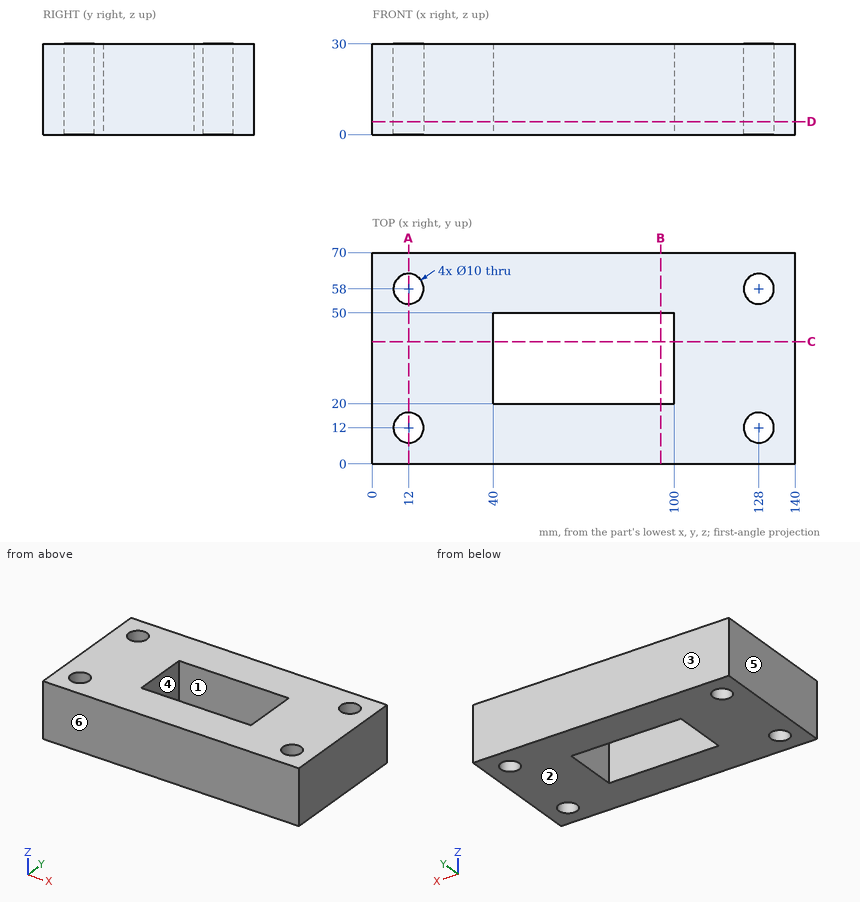
The drawing under review shows one solid part. Ordinate dimensions are in mm from its lowest x, y, z. A direction names the side the tool comes from. Give positions to 0.01 mm unless a question says otherwise; leave off trailing zeros. Write each loop counter-clockwise with the first axis right and the second up, starting at its lowest first coordinate (ties: lowest second). Pieces come first, ordered by that corner, then holes. Notation, with made-up numbers: (13, 20) -> (50, 20) arc R20 ccw to (50, 58) -> close; hole circle Ø8 at (6, -33). An arc over 180 degrees is marked (long way). Put each result on its own line as item: value.
(1) We need section B-B, the plane x = 95.5. Give the boundary of the cut face in (y, z), and give its area (3 significant figures).
Results are:
outline: (0, 0) -> (20, 0) -> (20, 30) -> (0, 30) -> close; (50, 0) -> (70, 0) -> (70, 30) -> (50, 30) -> close
area: 1,200 mm²
(2) We need section A-A, the plane x = 12. Give the boundary of the cut face in (y, z).
Results are:
outline: (0, 0) -> (7, 0) -> (7, 30) -> (0, 30) -> close; (17, 0) -> (53, 0) -> (53, 30) -> (17, 30) -> close; (63, 0) -> (70, 0) -> (70, 30) -> (63, 30) -> close
(3) The part is to be moulded in two halves that separate along Y. For the marked faces 3, 4, 5 and 6, say which applies: pulls with the +Y half, pulls with the -Y half, needs draft (parallel to the pull), parting line crosses it, or undercut.
Results are:
face 3: pulls with the +Y half
face 4: undercut
face 5: needs draft
face 6: pulls with the -Y half
(4) We need section C-C, the plane y = 40.5. Give the boundary of the cut face in (x, z), and give its area (3 significant figures).
Results are:
outline: (0, 0) -> (40, 0) -> (40, 30) -> (0, 30) -> close; (100, 0) -> (140, 0) -> (140, 30) -> (100, 30) -> close
area: 2,400 mm²
(5) For pin 1 Ø12 at (x, y) = (68, 42.5) entering from -Z, flat-tipped, find the tip position at first contact; note if it passes through.
Results are:
pin 1: through
(6) We need section D-D, the plane z = 4.25. Give the boundary of the cut face in (x, y).
Results are:
outline: (0, 0) -> (140, 0) -> (140, 70) -> (0, 70) -> close; hole circle Ø10 at (12, 12); hole circle Ø10 at (12, 58); hole (40, 20) -> (100, 20) -> (100, 50) -> (40, 50) -> close; hole circle Ø10 at (128, 12); hole circle Ø10 at (128, 58)
(7) To check wall thickness, follow probe 1 along Y at (x, z) = (128, 13); probe 2 along Y at (x, z) = (74.5, 10); probe 3 along Y at (x, z) = (11, 28). State the ranges of each line that lie inside material, in increasing order. Write a range as from..to.
Results are:
probe 1: 0..7, 17..53, 63..70
probe 2: 0..20, 50..70
probe 3: 0..7.1, 16.9..53.1, 62.9..70
(8) Tool access review of the marked faces 1 and 2: name each direction out of +Z, -Z, +X, -X, +Y, -Y from which nothing blocks a thin tool from reaching the whole face with its end or side.
Results are:
face 1: +Z, -Z
face 2: -Z, +X, -X, +Y, -Y
